Answer from the drawing. Dimensions are ordinates in mm from the lowest x, y and z of the part. Coordinates: 2 decimals unless noted, no trailing zeros. Loops run counter-clockwise (first coordinate to the right, second up) from the corner with the lowest first, then second, coordinate; pieces in that order, holes last. Notation, with made-up numbers: (-11.75, 28) - (-2.75, 28) arc R15 cw to (-2.75, 33) - close; hole circle Ø6 at (-17, -15). An arc over 180 degrees is marked (long way). Use one line per item in the form item = value. Start each with the question number.
1) A cutting plane is placed at B-B (y = 38.1). Give the vertices of the cut face in (x, z), and give its area (3 significant figures).
2) A cutting plane is placed at D-D (x = 50). Give the vertices of the cut face in (y, z), and give its area (3 significant figures).
3) This flat-tipped pin is pushed along its axis until it touches: P1, Ø12, axis at x = 38.1, y = 38.1, coming from the -Z side. Where does it stop, or does it pass through?
4) A cutting plane is placed at A-A (z = 38.1). Give the vertices of the cut face in (x, y), and give its area (3 significant figures).
5) The mould has two halves that part along Y. Classify the marked faces 1, 2 and 3: released by +Y, released by -Y, zero draft, split by the parting line, or undercut.
6) Consider line 1 (Y direction, x = 38, z = 59); line 2 (X direction, y = 39.5, z = 55). Determine where each line is inside the solid, lowest interval first.
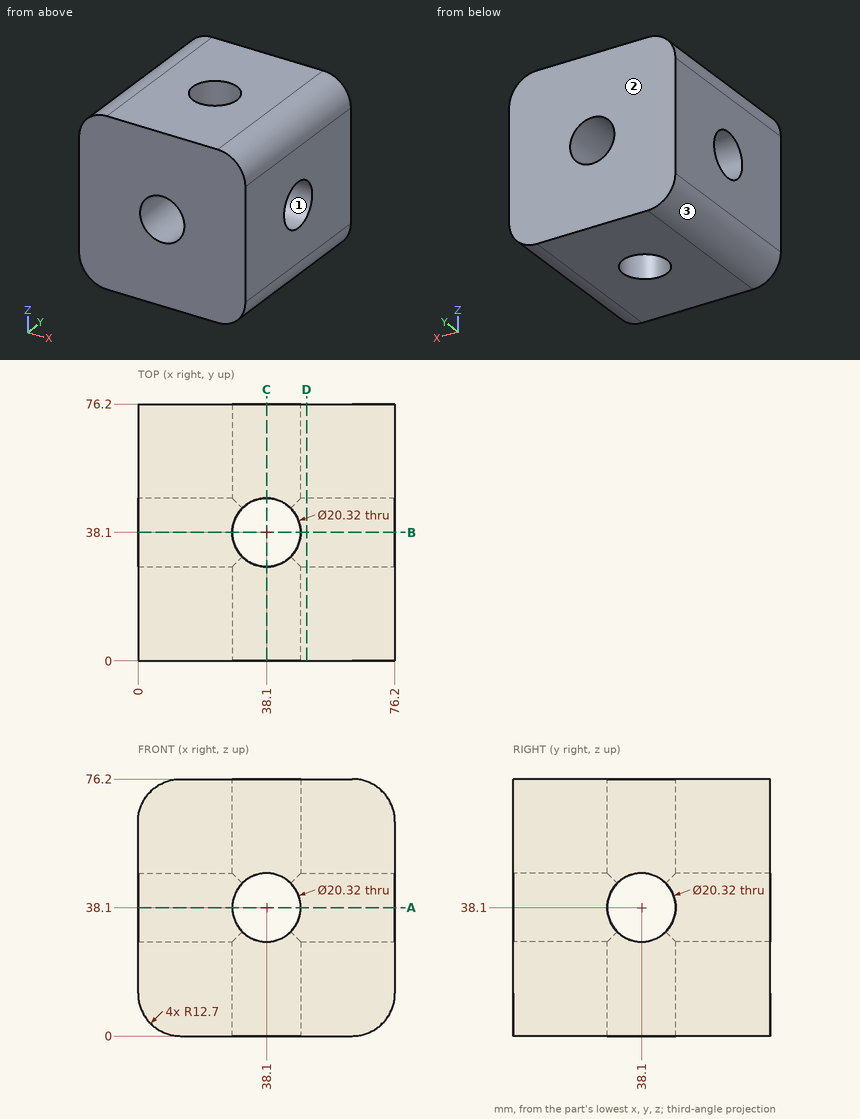
Found:
q1.outline = (0, 12.7) arc R12.7 ccw to (12.7, 0) - (27.94, 0) - (27.94, 27.94) - (0, 27.94) - close; (0, 48.26) - (27.94, 48.26) - (27.94, 76.2) - (12.7, 76.2) arc R12.7 ccw to (0, 63.5) - close; (48.26, 0) - (63.5, 0) arc R12.7 ccw to (76.2, 12.7) - (76.2, 27.94) - (48.26, 27.94) - close; (48.26, 48.26) - (76.2, 48.26) - (76.2, 63.5) arc R12.7 ccw to (63.5, 76.2) - (48.26, 76.2) - close
q1.area = 2,980 mm^2
q2.outline = (0, 0) - (76.2, 0) - (76.2, 76.2) - (0, 76.2) - close; hole circle Ø20.32 at (38.1, 38.1)
q2.area = 5,480 mm^2
q3.P1 = through
q4.outline = (0, 0) - (27.94, 0) - (27.94, 27.94) - (0, 27.94) - close; (0, 48.26) - (27.94, 48.26) - (27.94, 76.2) - (0, 76.2) - close; (48.26, 0) - (76.2, 0) - (76.2, 27.94) - (48.26, 27.94) - close; (48.26, 48.26) - (76.2, 48.26) - (76.2, 76.2) - (48.26, 76.2) - close
q4.area = 3,120 mm^2
q5.face_1 = undercut
q5.face_2 = released by +Y
q5.face_3 = zero draft
q6.line_1 = 0 to 27.94, 48.26 to 76.2
q6.line_2 = 0 to 28.04, 48.16 to 76.2
